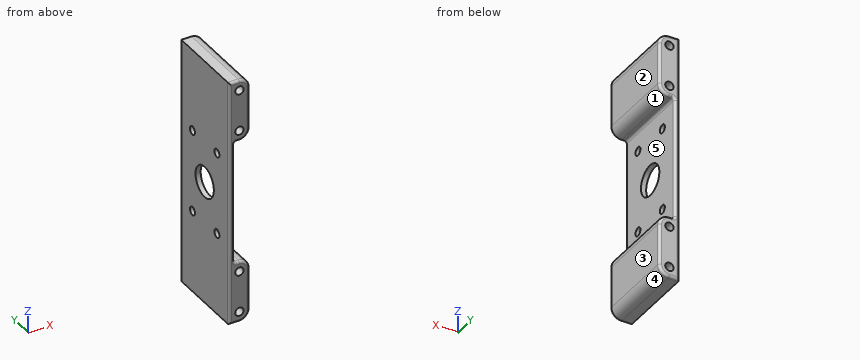
Autodesk Inventor part; units mm, degrees
ref_plane "YZ Plane" through (0, 0, 0) normal (1, 0, 0) x (0, 1, 0)
ref_plane "XZ Plane" through (0, 0, 0) normal (0, 1, 0) x (-1, 0, 0)
ref_plane "XY Plane" through (0, 0, 0) normal (0, 0, 1) x (1, 0, 0)
sketch "Sketch1" plane through (0, 0, 0) normal (0, 1, 0) x (-1, 0, 0)
  line L0 (0, 0) -> (-3.175, 0)
  line L1 (-3.175, 0) -> (-3.175, 101.6)
  line L2 (-3.175, 101.6) -> (0, 101.6)
  line L3 (0, 101.6) -> (0, 0)
  line L4 (0, 0) -> (-3.175, 0)
  line L5 (-3.175, 0) -> (-3.175, -25.4)
  line L6 (-3.175, -25.4) -> (0, -25.4)
  line L7 (0, -25.4) -> (0, 0)
  line L8 (0, 101.6) -> (-3.175, 101.6)
  line L9 (-3.175, 101.6) -> (-3.175, 127)
  line L10 (-3.175, 127) -> (0, 127)
  line L11 (0, 127) -> (0, 101.6)
  circle A0 centre (-6.35, 120.65) radius 2.5797
  circle A1 centre (-6.35, 95.25) radius 2.5797
  line L12 (0, 127) -> (-12.7, 127)
  line L13 (-12.7, 127) -> (-12.7, 88.9)
  line L14 (-12.7, 88.9) -> (0, 88.9)
  line L15 (0, 88.9) -> (0, 127)
  line L16 (25.4, 50.8) -> (-25.4, 50.8)
  line L17 (25.4, 50.8) -> (76.2, 50.8) construction
  line L18 (-3.175, 101.6) -> (-3.175, 0)
  line L19 (-3.175, 0) -> (0, 0)
  line L20 (0, 0) -> (0, 101.6)
  line L21 (0, 0) -> (-3.175, 0)
  line L22 (-3.175, 0) -> (-3.175, -25.4)
  line L23 (-3.175, -25.4) -> (0, -25.4)
  line L24 (0, -25.4) -> (0, 0)
  circle A2 centre (-6.35, -19.05) radius 2.5797
  circle A3 centre (-6.35, 6.35) radius 2.5797
  line L25 (0, -25.4) -> (-12.7, -25.4)
  line L26 (-12.7, -25.4) -> (-12.7, 12.7)
  line L27 (-12.7, 12.7) -> (0, 12.7)
  line L28 (0, 12.7) -> (0, -25.4)
  circle A4 centre (-6.35, 6.35) radius 6.35
  circle A5 centre (-6.35, -19.05) radius 6.35
  circle A6 centre (-6.35, 95.25) radius 6.35
  circle A7 centre (-6.35, 120.65) radius 6.35
  point P0 (-3.175, 88.9)
  point P1 (-3.175, 12.7)
  point P2 (-12.7, -19.05)
  point P3 (0, -19.05)
  point P4 (0, 120.65)
  point P5 (-3.175, 115.1507)
  point P6 (-3.175, 100.7493)
  point P7 (-6.35, 88.9)
  point P8 (-6.35, 12.7)
  point P9 (-12.7, 6.35)
  point P10 (-6.35, 127)
  point P11 (-12.7, 120.65)
  point P12 (-12.7, 95.25)
  point P13 (-6.35, -25.4)
  dimension "d25" = 3.175
  dimension "d26" = 101.6
  dimension "d27" = 3.175
  dimension "d28" = 25.4
  dimension "d29" = 3.175
  dimension "d30" = 25.4
  dimension "d31" = 0
  dimension "d32" = 25.4
  dimension "d33" = 6.35
  dimension "d34" = 5.1594
  dimension "d35" = 5.1594
  dimension "d36" = 12.7
  dimension "d37" = 38.1
  dimension "d38" = 6.35
  dimension "d39" = 50.8
  dimension "d40" = 180
  dimension "d41" = 50.8
  dimension "d42" = 25.4
extrude "Extrusion1" add sketch "Sketch1" along normal blind 50.8 contours L7 A5 L5 L0 | L0 L1 A4 L3 | L5 A5 L26 A4 L1 | A4 L1 L27 L3 | A4 L1 | A5 L5 | L7 L6 L5 A5 | A4 L1 | L5 A5 | L27 L1 L16 L3 | A4 L27 L1 | L5 L25 A5 | L16 L1 L14 L3 | L14 L1 A6 L3 | A6 L1 L2 L3 | A6 L1 | L14 A6 L1 | L2 L9 A7 L11 | A6 L13 A7 L9 L1 | L1 A6 | A7 L9 L10 L11 | A7 L9 | A7 L9 | A7 L12 L9
sketch "Sketch3" plane through (3.175, 0, 88.9) normal (1, 0, 0) x (0, 0, -1)
  circle A0 centre (12.7, 12.7) radius 2.5797
  line L0 (0, 0) -> (76.2, 0)
  line L1 (0, 0) -> (0, 50.8)
  circle A1 centre (63.5, 12.7) radius 2.5797
  circle A2 centre (12.7, 38.1) radius 2.5797
  circle A3 centre (63.5, 38.1) radius 2.5797
  circle A4 centre (38.1, 25.4) radius 9.525
  point P0 (88.9, 0)
  dimension "d43" = 12.7
  dimension "d44" = 12.7
  dimension "d45" = 5.1594
  dimension "d48" = 50.8
  dimension "d51" = 25.4
  dimension "d56" = 19.05
  dimension "d57" = 25.4
  dimension "d58" = 38.1
extrude "Extrusion3" cut sketch "Sketch3" against normal blind 50.8
fillet "Fillet3" radius 1.5875 26 edges at (0, 50.8, 50.8) (0, 0, 50.8) (10.8401, 50.8, 125.1401) (12.7, 50.8, 107.95) (10.8401, 50.8, 90.7599) (4.7625, 50.8, 88.9) (3.175, 50.8, 127) (10.8401, 0, 125.1401) (12.7, 0, 107.95) (10.8401, 0, 90.7599) (4.7625, 0, 88.9) (3.175, 0, 127) (3.175, 25.4, 88.9) (3.175, 50.8, 50.8) (3.175, 50.8, -25.4) (12.7, 50.8, -6.35) (10.8401, 50.8, 10.8401) (4.7625, 50.8, 12.7) (10.8401, 50.8, -23.5401) (3.175, 0, -25.4) (12.7, 0, -6.35) (10.8401, 0, 10.8401) (4.7625, 0, 12.7) (10.8401, 0, -23.5401) (3.175, 0, 50.8) (3.175, 25.4, 12.7)
equation "\"d35\" = d34"
properties part number "Connector plate"
Here's how the part is built. I have some questions about the finished solid (model axes, mm). Face numbers are marked on the shaded views. A direction names the side the tool comes from. Coordinates: 2 decimals unless noted, no trailing zeros. Order: outer loops, then holes, each group sorted by start corner. A loop starts at its lowest first (then second) coordinate and runs counter-clockwise, first axis right, second up.
Item 1: Thinking about a two-plate mould opening in Z: for the marked faces 3, 4 and 5, which applies, pulls with the +Z half, pulls with the -Z half, needs draft (parallel to the pull), parting line crosses it, or undercut?
Response values:
face 3: needs draft
face 4: pulls with the -Z half
face 5: undercut
Item 2: Which directions (+Z, -Z, +X, -X, +Y, -Y) give clear straight access to the entire face, cutting with the end or side of a thin tool? Please do the marked faces 1 and 2.
Response values:
face 1: +X, +Y, -Y
face 2: +Z, -Z, +X, +Y, -Y
Item 3: I'm going to push flat-ended pins straight in: pin 1 Ø1.5 at (x, y) = (9.5, 18.5) entering from +Z; pin 2 Ø3 at (y, z) = (12.7, 76.2) entering from -X; pin 3 Ø5 at (y, z) = (11, 87) entering from +X. Where does each tip first touch, or does it pass through?
Response values:
pin 1: stops at z = 126.53
pin 2: passes through
pin 3: stops at x = 9.04
Item 4: I need wall thicknesses on probe 1 along Z at (x, y) = (6.35, 31.5); probe 2 along Z at (x, y) = (7.25, 33.5); probe 3 along Y at (x, z) = (0.85, 25.4). Which ranges of each line are inside material? Lowest first, please.
Response values:
probe 1: z = -25.4 to -21.63, -16.47 to 3.77, 8.93 to 12.7, 88.9 to 92.67, 97.83 to 118.07, 123.23 to 127
probe 2: z = -25.34 to -21.47, -16.63 to 3.93, 8.77 to 12.64, 88.96 to 92.83, 97.67 to 118.23, 123.07 to 126.94
probe 3: y = 0.18 to 10.12, 15.28 to 35.52, 40.68 to 50.62
Item 5: If we section it at D-D, the plane z = 76.2: Give the number of separate pieces and of enclosed holes in the cut face, then the cut area to 3 significant figures.
Response values:
separate pieces: 3
enclosed holes: 0
area: 126 mm2
Item 6: If we section it at C-C, the plane y = 31.5: List the corners of the cut face in (x, z) for me (3 decimals).
Response values:
outline: (0, -25.4) - (6.35, -25.4) arc R6.35 ccw to (12.7, -19.05) - (12.7, 6.35) arc R6.35 ccw to (6.35, 12.7) - (4.762, 12.7) arc R1.587 cw to (3.175, 14.287) - (3.175, 43.485) - (0, 43.485) - close; (0, 58.115) - (3.175, 58.115) - (3.175, 87.313) arc R1.587 cw to (4.762, 88.9) - (6.35, 88.9) arc R6.35 ccw to (12.7, 95.25) - (12.7, 120.65) arc R6.35 ccw to (6.35, 127) - (0, 127) - close; hole circle Ø5.159 at (6.35, -19.05); hole circle Ø5.159 at (6.35, 6.35); hole circle Ø5.159 at (6.35, 95.25); hole circle Ø5.159 at (6.35, 120.65)
Item 7: If we section it at A-A, the plane y = 38.1: List the corners of the cut face in (x, z) for me (3 decimals), then the cut area to 3 significant figures.
Response values:
outline: (0, -25.4) - (6.35, -25.4) arc R6.35 ccw to (12.7, -19.05) - (12.7, 6.35) arc R6.35 ccw to (6.35, 12.7) - (4.762, 12.7) arc R1.587 cw to (3.175, 14.287) - (3.175, 22.82) - (0, 22.82) - close; (0, 27.98) - (3.175, 27.98) - (3.175, 73.62) - (0, 73.62) - close; (0, 78.78) - (3.175, 78.78) - (3.175, 87.313) arc R1.587 cw to (4.762, 88.9) - (6.35, 88.9) arc R6.35 ccw to (12.7, 95.25) - (12.7, 120.65) arc R6.35 ccw to (6.35, 127) - (0, 127) - close; hole circle Ø5.159 at (6.35, -19.05); hole circle Ø5.159 at (6.35, 6.35); hole circle Ø5.159 at (6.35, 95.25); hole circle Ø5.159 at (6.35, 120.65)
area: 1,060 mm2
